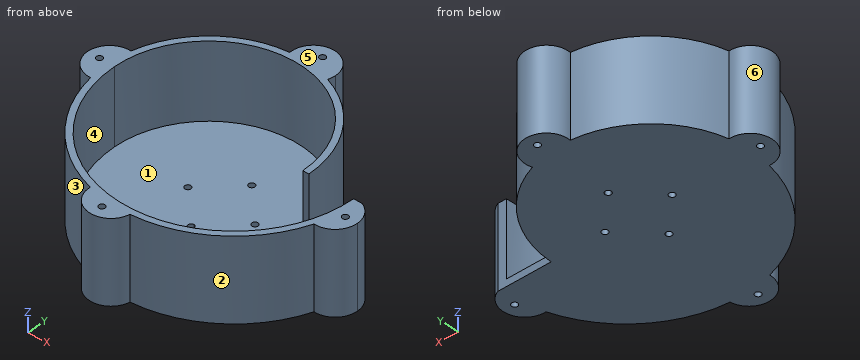
```python
from build123d import *

# Parameters (mm, degrees)
F0_R     = 40
F1_DEPTH = 3.5
F2_DEPTH = 37
F3_R     = 1.5
F4_DEPTH = 25
F5_R     = 1.5
F6_DEPTH = 40.5


with BuildPart() as f1:
    # F0 (on Top) → F1 (new body)
    with BuildSketch(Plane.XY):
        with BuildLine():
            Line((43, 0), (40, 0))
            ThreePointArc((40, 0), (-6.25, 46.25), (-52.5, 0))
            ThreePointArc((-52.5, 0), (6.25, -58.75), (65, 0))
            Line((65, 0), (43, 0))
        make_face()
        Circle(F0_R, mode=Mode.SUBTRACT)
        Circle(F0_R)
        with BuildLine():
            ThreePointArc((-52.5, 0), (-6.25, 46.25), (40, 0))
            Line((40, 0), (43, 0))
            ThreePointArc((43, 0), (-6.25, 49.25), (-55.5, 0))
            ThreePointArc((-55.5, 0), (6.25, -61.75), (68, 0))
            Line((68, 0), (65, 0))
            ThreePointArc((65, 0), (6.25, -58.75), (-52.5, 0))
        make_face()
    extrude(amount=-F1_DEPTH)

    # F0 (on Top) → F2 (join)
    with BuildSketch(Plane.XY):
        with BuildLine():
            ThreePointArc((-52.5, 0), (-6.25, 46.25), (40, 0))
            Line((40, 0), (43, 0))
            ThreePointArc((43, 0), (-6.25, 49.25), (-55.5, 0))
            ThreePointArc((-55.5, 0), (6.25, -61.75), (68, 0))
            Line((68, 0), (65, 0))
            ThreePointArc((65, 0), (6.25, -58.75), (-52.5, 0))
        make_face()
    extrude(amount=F2_DEPTH)

    # F3 (on face) → F4 (cut)
    with BuildSketch(Plane.XY):
        with BuildLine():
            ThreePointArc((1.5, 16.5), (-1.0606601718, 17.5606601718), (0, 15))
            ThreePointArc((0, 15), (1.0606601718, 15.4393398282), (1.5, 16.5))
        make_face()
        with BuildLine():
            ThreePointArc((18, 0), (16.5, 1.5), (15, 0))
            ThreePointArc((15, 0), (16.5, -1.5), (18, 0))
        make_face()
        with BuildLine():
            ThreePointArc((1.5, -16.5), (1.0606601718, -15.4393398282), (0, -15))
            ThreePointArc((0, -15), (-1.0606601718, -17.5606601718), (1.5, -16.5))
        make_face()
        with Locations((-16.5, 0)):
            Circle(F3_R)
    extrude(amount=-F4_DEPTH, mode=Mode.SUBTRACT)

    # F5 (on face) → F6 (join)
    with BuildSketch(Plane(origin=(0, 0, -3.5), x_dir=(1, 0, 0), z_dir=(0, 0, -1))):
        with BuildLine():
            ThreePointArc((10.7428359613, 61.5863371619), (-1.1250923825, 70.8008868716), (-10.8391434064, 59.3382143111))
            ThreePointArc((-10.8391434064, 59.3382143111), (-0.147675703, 61.417686749), (10.7428359613, 61.5863371619))
        make_face()
        with Locations((0, 65)):
            Circle(F5_R, mode=Mode.SUBTRACT)
        with BuildLine():
            ThreePointArc((-55.5, 0), (-55.2593781422, 5.4459985826), (-54.5393878361, 10.8495542082))
            ThreePointArc((-54.5393878361, 10.8495542082), (-65.8586269328, -0.1233337651), (-54.2930770248, -10.8362931849))
            ThreePointArc((-54.2930770248, -10.8362931849), (-55.1973392713, -5.4516491325), (-55.5, 0))
        make_face()
        with Locations((-60, 0)):
            Circle(F5_R, mode=Mode.SUBTRACT)
        with BuildLine():
            ThreePointArc((10.2469559678, -46.4048806032), (-0.1412893215, -48.8696854281), (-10.8166174818, -49.0378272844))
            ThreePointArc((-10.8166174818, -49.0378272844), (-0.481560086, -60.8486446142), (10.859327331, -50))
            ThreePointArc((10.859327331, -50), (10.7051398656, -48.1765498249), (10.2469559678, -46.4048806032))
        make_face()
        with Locations((0, -55)):
            Circle(F5_R, mode=Mode.SUBTRACT)
        with BuildLine():
            ThreePointArc((75.859327331, 10), (72.4550295609, 17.8960448535), (64.3765674089, 20.8414169686))
            ThreePointArc((64.3765674089, 20.8414169686), (67.0873981918, 10.5770261061), (68, 0))
            Line((68, 0), (69.2337914548, 0))
            ThreePointArc((69.2337914548, 0), (74.0526547858, 4.0021310941), (75.859327331, 10))
        make_face()
        with Locations((70, 10)):
            Circle(F5_R, mode=Mode.SUBTRACT)
    extrude(amount=-F6_DEPTH)


solid = f1.part
```
Could you check a few things on this model? Use its own coordinates, in mm. Face numbers are marked on the shaded views. A direction names the side the tool comes from. Give positions to 0.01 mm unless a question says otherwise; leave off trailing zeros. Write each loop counter-clockwise with the first axis right and the second up, starting at its lowest first coordinate (ties: lowest second). Pieces come first, ordered by that corner, then holes. Notation, with made-up numbers: (44, 10.25) - (71, 10.25) arc R30 ccw to (71, 32.25) - close; hole circle Ø4 at (39.25, -32). An arc over 180 degrees is marked (long way). One line per item, written item: value. Start each with the question number.
Item 1: Imagine slicing it at A-A, the plane z = 5. List the corners of the cut face in (x, y) for me, and give its area (3 significant figures).
Item 2: Imagine slicing it at C-C, the plane x = -41. List the corners of the cut face in (y, z) for me.
Item 3: If we mould it in two halves opening along Y, with no side actions, what happens to the marked faces 3, 4, 5 and 6? For each: +Y half, -Y half, draft (parallel to the pull), parting line (faces both ways), or undercut.
Item 4: Which directions (+Z, -Z, +X, -X, +Y, -Y) give clear straight access to the entire face, cutting with the end or side of a thin tool? Please do the marked faces 1 and 2.
Item 5: Imagine slicing it at B-B, the plane y = 24. List the corners of the cut face in (x, z) for me.
Item 6: I'm going to push flat-ended pins straight in: pin 1 (1.5 mm diameter, centred on x = 41, z = 27, fed in from -Y); pin 2 (3 mm diameter, centred on y = 31, z = 31, fed in from -X); pin 3 (3.5 mm diameter, centred on x = -16.5, y = 0, fed in from +Z). Where does each tip first touch, or does it pass through?
Item 7: Please list where these lines run through material, in increasing order: line 1 (Y direction, x = 0, z = 24); line 2 (Z direction, x = 57.5, y = -4); line 3 (X direction, y = -19, z = 5). Write a range as from..to.
Geometry says:
1. outline: (-54.54, -10.85) arc R61.75 ccw to (-10.84, -59.34) arc R10.86 ccw to (10.74, -61.59) arc R61.75 ccw to (64.38, -20.84) arc R10.86 ccw to (69.23, 0) - (65, 0) arc R58.75 cw to (-52.5, 0) arc R46.25 cw to (40, 0) - (43, 0) arc R49.25 ccw to (10.25, 46.4) arc R10.86 ccw (long way) to (-10.82, 49.04) arc R49.25 ccw to (-54.29, 10.84) arc R10.86 ccw (long way) to start; hole circle Ø3 at (-60, 0); hole circle Ø3 at (0, -65); hole circle Ø3 at (0, 55); hole circle Ø3 at (70, -10)
1. area: 1,700 mm^2
2. outline: (-39.76, -3.5) - (34.9, -3.5) - (34.9, 37) - (30.52, 37) - (30.52, 0) - (-34.91, 0) - (-34.91, 37) - (-39.76, 37) - close
3. face 3: -Y half
3. face 4: undercut
3. face 5: draft
3. face 6: parting line
4. face 1: +Z
4. face 2: +Z, -Z, +X, -Y
5. outline: (-49.26, -3.5) - (36.76, -3.5) - (36.76, 37) - (33.29, 37) - (33.29, 0) - (-45.79, 0) - (-45.79, 37) - (-49.26, 37) - close
6. pin 1: y = -51.55
6. pin 2: x = -45.69
6. pin 3: z = 0
7. line 1: -70.86..-66.5, -63.5..-58.42, 45.83..53.5, 56.5..60.86
7. line 2: -3.5..0
7. line 3: -52.5..-49.34, 61.84..71.08
